Autodesk Inventor part; units mm, degrees
ref_plane "YZ Plane" through (0, 0, 0) normal (1, 0, 0) x (0, 1, 0)
ref_plane "XZ Plane" through (0, 0, 0) normal (0, 1, 0) x (-1, 0, 0)
ref_plane "XY Plane" through (0, 0, 0) normal (0, 0, 1) x (1, 0, 0)
sketch "Sketch1" plane through (0, 0, 0) normal (0, 1, 0) x (-1, 0, 0)
  line L0 (-18.2563, -12.5) -> (18.2563, -12.5)
  line L1 (18.2563, -12.5) -> (18.2563, 12.5)
  line L2 (18.2563, 12.5) -> (-18.2563, 12.5)
  line L3 (-18.2563, 12.5) -> (-18.2563, -12.5)
  line L4 (-18.2563, -12.5) -> (18.2563, 12.5) construction
  line L5 (18.2563, -12.5) -> (-18.2563, 12.5) construction
  point P0 (0, 0)
  dimension "d0" = 36.5125
  dimension "d1" = 25
extrude "Extrusion1" add sketch "Sketch1" against normal blind 5
sketch "Sketch2" plane through (18.2563, 0, 12.5) normal (1, 0, 0) x (0, 0, -1)
  line L0 (25, 0) -> (25, -5)
  circle A0 centre (30, 0) radius 5
  line L1 (25, -5) -> (0, -5)
  line L2 (25, -5) -> (30, -5)
  line L3 (30, -5) -> (30, 0)
  line L4 (30, 0) -> (25, 0)
  line L5 (25, 0) -> (25, -5)
  point P0 (12.5, 0)
  dimension "d4" = 5
  dimension "d5" = 5
extrude "Extrusion2" add sketch "Sketch2" against normal blind 36.513
sketch "Sketch3" plane through (18.2563, -5, 12.5) normal (1, 0, 0) x (0, 0, -1)
  circle A0 centre (30, 5) radius 2.5
  line L0 (0, 5) -> (25, 5)
  point P0 (12.5, 5)
  dimension "d8" = 0
  dimension "d9" = 5
  dimension "d10" = 5
extrude "Extrusion3" cut sketch "Sketch3" against normal blind 36.513
sketch "Sketch4" plane through (0, -5, 0) normal (0, -1, 0) x (1, 0, 0)
  line L0 (18.2563, -12.5) -> (-18.2563, -12.5)
  line L1 (18.2563, -22.5) -> (-18.2567, -22.5)
  line L2 (8.2563, -12.5) -> (-8.2568, -12.5)
  line L3 (-8.2568, -12.5) -> (-8.2567, -22.5)
  line L4 (-8.2567, -22.5) -> (8.2563, -22.5)
  line L5 (8.2563, -22.5) -> (8.2563, -12.5)
  line L6 (18.2563, -22.5) -> (18.2563, -12.5)
  line L7 (-18.2567, -12.5) -> (-18.2567, -22.5)
  line L8 (8.2563, -12.5) -> (-8.2567, -12.5)
  line L9 (-8.2567, -12.5) -> (-8.2567, -9.5)
  line L10 (-8.2567, -9.5) -> (8.2562, -9.5)
  line L11 (8.2562, -9.5) -> (8.2563, -12.5)
  point P0 (0, 0)
  point P1 (18.2563, -17.5)
  point P2 (-18.2567, -17.5)
  point P3 (8.2562, -11)
  dimension "d13" = 10
  dimension "d14" = 10
  dimension "d15" = 3
  dimension "d16" = 16.513
extrude "Extrusion4" cut sketch "Sketch4" against normal blind 36.513 contours L5 L1 L3 L0 | L0 L9 L10 L11
properties part number "hinge 1" material "Stainless Steel"
Geometry check sheet. Reference: the model listing, model coordinates, mm. A direction names the side the tool comes from. Coordinates: 2 decimals unless noted, no trailing zeros. Order: outer loops, then holes, each group sorted by start corner. A loop starts at its lowest first (then second) coordinate and runs counter-clockwise, first axis right, second up. Notation, with made-up numbers: (86, 78.5) - (101, 78.5) arc R29 cw to (101, 114.5) - close; hole circle Ø7 at (-37.75, 34). An arc over 180 degrees is marked (long way). Use one line per item in the form item = value.
1. Draft check along Y on faces 4 (the face through (13, 0, -15)), 5 (the face through (-13.19, 3.42, -21.15)), 6 (the face through (-18.256, -2, 0)). Enter one of: pulls with the +Y half, pulls with the -Y half, needs draft (parallel to the pull), parting line crosses it, or undercut.
Here are the results:
face_4 = undercut
face_5 = parting line crosses it
face_6 = needs draft
2. Scan lines: line 1 (Y direction, x = -14.75, z = -17.5); line 2 (Y direction, x = 16.5, z = 7.5); line 3 (X direction, y = -2.5, z = -15.5). Record each from-to range of solid material in increasing order.
Here are the results:
line_1 = -5 to -2.5, 2.5 to 5
line_2 = -5 to 0
line_3 = -18.26 to -8.26, 8.26 to 18.26
3. Access from +Z, -Z, +X, -X, +Y, -Y to the whole of each face (thin tool, end or side, straight path). Record for faces 1 (the face through (0, 0, 0)), 2 (the face through (0, -5, -2)), 3 (the face through (0, -3, -9.5)).
Here are the results:
face_1 = +Z, +X, -X, +Y
face_2 = +Z, -Z, +X, -X, -Y
face_3 = -Z, +Y, -Y
4. Section check B-B (z = -11). Record the boundary of the cut face in (x, y).
Here are the results:
outline = (-18.26, -5) - (-8.26, -5) - (-8.26, 0) - (-18.26, 0) - close; (8.26, -5) - (18.26, -5) - (18.26, 0) - (8.26, 0) - close
5. Section check D-D (x = -9). Record the boundary of the cut face in (y, z), then the cut area to 3 significant figures.
Here are the results:
outline = (-5, -17.5) arc R5 ccw (long way) to (0, -12.5) - (0, 12.5) - (-5, 12.5) - close; hole circle Ø5 at (0, -17.5)
area = 189 mm²
6. Section check A-A (y = 4). Record the boundary of the cut face in (x, z), then the cut area to 3 significant figures.
Here are the results:
outline = (-18.26, -20.5) - (-8.26, -20.5) - (-8.26, -14.5) - (-18.26, -14.5) - close; (8.26, -20.5) - (18.26, -20.5) - (18.26, -14.5) - (8.26, -14.5) - close
area = 120 mm²
7. Gauge pin test, flat ends, axial feed: pin 1 (1.5 mm diameter, centred on x = -1, y = -3.5, fed in from -Z); pin 2 (3 mm diameter, centred on x = -12.5, z = -2.5, fed in from +Y); pin 3 (4.5 mm diameter, centred on y = 0, z = -17.5, fed in from -X). Record the tip position at first contact, or that the pin passes through.
Here are the results:
pin_1 = -9.5
pin_2 = 0
pin_3 = through
